Study the drawing (mm; zero at the part's minimum x, y, z) and answer. A direction names the side the tool comes from. Coordinates: 2 decimals unless noted, no trailing zeros. Order: outer loops, then holes, each group sorted by start corner. A loop starts at its lowest first (then second) coordinate and runs counter-clockwise, first axis right, second up. Notation, with made-up numbers: M 89.5,3.5 L 117.5,3.5 A5 cw 117.5,9.5 Z; hole C -32.75,-19 d5. An arc over 180 degrees is marked long. Use a Markdown table: item, result. Add a question column.
1) Find section C-C on z = 5.5. Write down the section's boundary in (x, y).
2) The mould has two halves that part along X. Classify the marked faces 4, 5 and 6: released by +X, released by -X, zero draft, split by the parting line, or undercut.
3) Find the intervals of material crossed by probe 1 along Z at (x, y) = (20, 0.85); probe 2 along X at (y, z) = (15, 20); probe 3 along Y at (x, z) = (13, 5), in increasing order. Write a range as [from, to].
4) Find section A-A on z = 20. Count the separate pieces of the cut face and the enclosed holes in it, plus the area to 3 significant figures.
5) Find section D-D on x = 33. Write down the section's boundary in (y, z).
6) For the marked faces 1, 2 and 3, determine the directions among +Z, -Z, +X, -X, +Y, -Y from which every point of the face is accessible in a straight line to the end or side of a thin tool.
7) Each of these flat-tipped pins is pushed along its axis until it touches: pin 1 Ø6 at (x, z) = (20, 5.5) entering from -Y; pin 2 Ø10 at (x, z) = (6, 13) entering from +Y; pin 3 Ø1.5 at (y, z) = (25, 25.5) entering from -X. Where does it stop, or does it pass through?
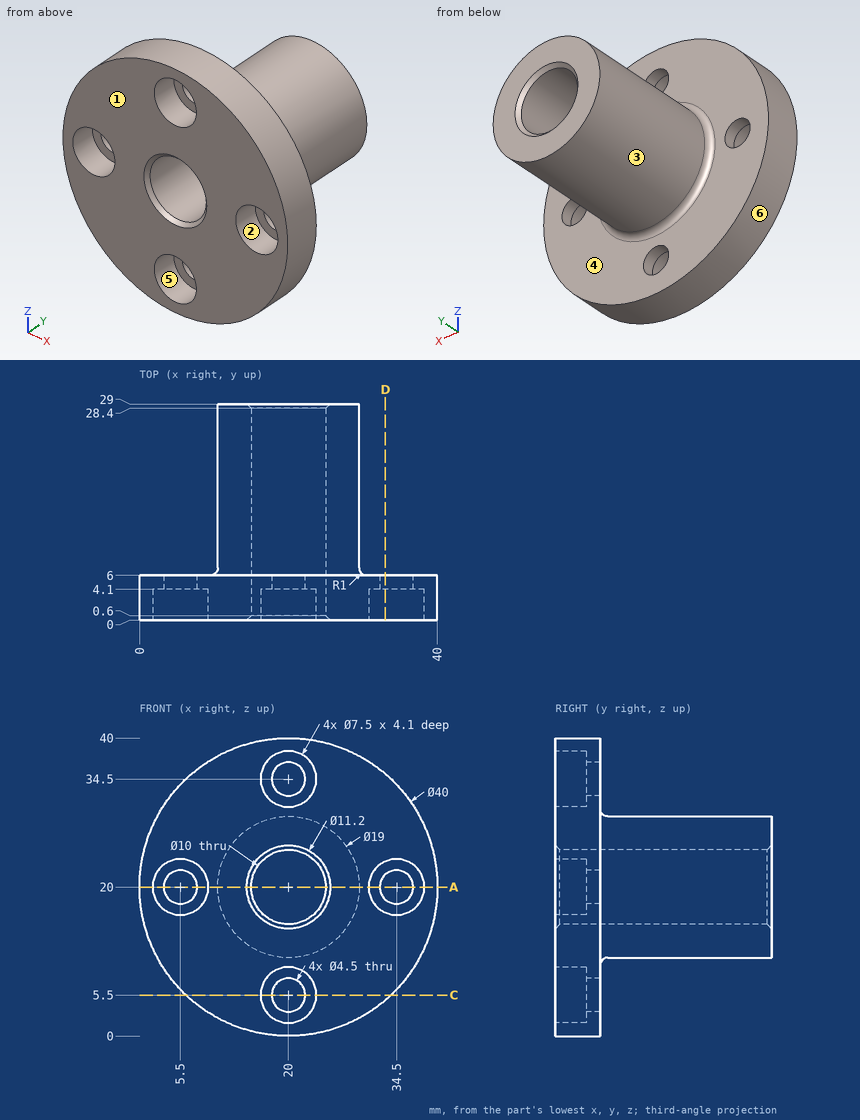
Check result:
| question | item | result |
|---|---|---|
| 1 | outline | M 6.23,0 L 16.25,0 L 16.25,4.1 L 17.75,4.1 L 17.75,6 L 6.23,6 Z; M 22.25,4.1 L 23.75,4.1 L 23.75,0 L 33.77,0 L 33.77,6 L 22.25,6 Z |
| 2 | face 4 | zero draft |
| 2 | face 5 | undercut |
| 2 | face 6 | split by the parting line |
| 3 | probe 1 | z = [0, 1.75], [9.25, 15], [25, 30.75], [38.25, 40] |
| 3 | probe 2 | x = [10.5, 15], [25, 29.5] |
| 3 | probe 3 | y = [0, 6] |
| 4 | separate pieces | 4 |
| 4 | enclosed holes | 0 |
| 4 | area | 308 mm2 |
| 5 | outline | M 0,4.8 L 6,4.8 L 6,18.32 L 4.1,18.32 L 4.1,16.56 L 0,16.56 Z; M 0,23.44 L 4.1,23.44 L 4.1,21.68 L 6,21.68 L 6,35.2 L 0,35.2 Z |
| 6 | face 1 | +Z, -Z, +X, -X, -Y |
| 6 | face 2 | -Y |
| 6 | face 3 | +Y |
| 7 | pin 1 | stops at y = 4.1 |
| 7 | pin 2 | stops at y = 6 |
| 7 | pin 3 | stops at x = 11.77 |
